Verification items for the finished model (mm, model axes). Face numbers are marked on the shaded views. A direction names the side the tool comes from. Round coordinates to 2 decimals unless told otherwise and drop trailing zeros. Write each loop counter-clockwise with the first axis right and the second up, starting at its lowest first coordinate (ties: lowest second). Pieces come first, ordered by that corner, then holes. Notation, with made-up numbers: (72.5, 87) -> (128.5, 87) arc R21 ccw to (128.5, 92) -> close; hole circle Ø2 at (9.5, 25). An arc over 180 degrees is marked (long way). Answer as a JSON object with one key per item and string values. Group by question number.
(1) Sectioned sample at A-A on x = 0. Record the cut outline in (y, z).
(2) Sectioned sample at B-B on z = 14.25. Record the cut outline in (x, y), and give its area (3 significant figures).
(3) Set-up check for the marked faces 1, 2, 3 and 4: record each of +Z, -Z, +X, -X, +Y, -Y from which the full face is reachable in a straight line by a thin tool's end or side.
(4) Gauge pin test, flat ends, axial feed: pin 1 Ø0.9 at (y, z) = (1, 23.5) entering from +X; pin 2 Ø2.5 at (x, y) = (0, 0) entering from +Z; pin 3 Ø1 at (x, z) = (-4, 18) entering from -Y. Record the tip position at first contact, or that the pin passes through.
(5) Sectioned sample at D-D on z = 5.25. Record the cut outline in (x, y), and give its area (3 significant figures).
(6) Scan lines: L1, parallel to X at y = 0, z = 16.75; L2, parallel to Z at x = -2.5, y = 6; L3, parallel to Y at x = -0.75, z = 12.75. Record each from-to range of solid material in increasing order. Write a range as from..to.
(7) Sectioned sample at C-C on y = 6.5. Record the cut outline in (x, z).
Solid Edge part; units mm, degrees
sketch "Sketch1" plane through (0, 0, 0) normal (0, 0, 1) x (1, 0, 0)
  circle A0 centre (0, 0) radius 15
extrude "Protrusion1" add sketch "Sketch1" along normal blind 10
sketch "Sketch2" plane through (0, 0, 10) normal (0, 0, 1) x (1, 0, 0)
  circle A0 centre (0, 0) radius 8
extrude "Extrusionsausprägung_2" add sketch "Sketch2" along normal blind 10
sketch "Sketch3" plane through (0, 0, 20) normal (0, 0, 1) x (1, 0, 0)
  circle A0 centre (0, 0) radius 6
extrude "Extrusionsausprägung_3" add sketch "Sketch3" along normal blind 2.5
sketch "Sketch4" plane through (0, 0, 22.5) normal (0, 0, 1) x (1, 0, 0)
  line L0 (-3.25, -3.25) -> (3.25, -3.25)
  line L1 (3.25, -3.25) -> (3.25, 3.25)
  line L2 (3.25, 3.25) -> (-3.25, 3.25)
  line L3 (-3.25, 3.25) -> (-3.25, -3.25)
extrude "Extrusionsausprägung_4" add sketch "Sketch4" along normal blind 3
sketch "Sketch5" plane through (0, 0, 10) normal (0, 0, 1) x (1, 0, 0)
  line L0 (-16.4348, 18.9803) -> (16.4348, 18.9803)
  line L1 (16.4348, 18.9803) -> (16.4348, -18.9803)
  line L2 (16.4348, -18.9803) -> (-16.4348, -18.9803)
  line L3 (-16.4348, -18.9803) -> (-16.4348, 18.9803)
  line L4 (-8, 16.4595) -> (8, 16.4595)
  line L5 (8, 16.4595) -> (8, -16.4595)
  line L6 (8, -16.4595) -> (-8, -16.4595)
  line L7 (-8, -16.4595) -> (-8, 16.4595)
  dimension "D1" = 8
extrude "Cutout1" cut sketch "Sketch5" against normal through all
hole "Bohrung_1" at (0, 0, 25.5) direction (0, 0, -1) diameter 3 depth 15
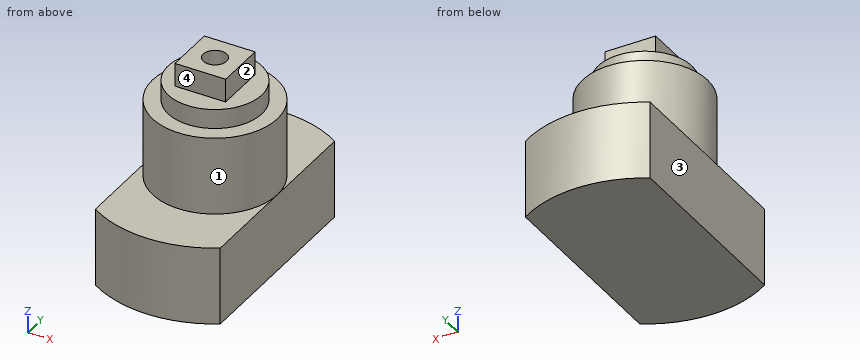
Computed values:
{
 "1": {"outline": "(-15, 0) -> (15, 0) -> (15, 10) -> (8, 10) -> (8, 20) -> (6, 20) -> (6, 22.5) -> (3.25, 22.5) -> (3.25, 25.5) -> (1.5, 25.5) -> (1.5, 10.5) -> (-1.5, 10.5) -> (-1.5, 25.5) -> (-3.25, 25.5) -> (-3.25, 22.5) -> (-6, 22.5) -> (-6, 20) -> (-8, 20) -> (-8, 10) -> (-15, 10) -> close"},
 "2": {"outline": "circle Ø16 at (0, 0); hole circle Ø3 at (0, 0)", "area": "194 mm2"},
 "3": {"face 1": "+Z", "face 2": "+Z, +X, +Y, -Y", "face 3": "+Z, -Z, -X, +Y, -Y", "face 4": "+Z, +X, -X, -Y"},
 "4": {"pin 1": "x = 3.25", "pin 2": "z = 10.5", "pin 3": "y = -7.19"},
 "5": {"outline": "(-8, -12.69) arc R15 ccw to (8, -12.69) -> (8, 12.69) arc R15 ccw to (-8, 12.69) -> close", "area": "456 mm2"},
 "6": {"L1": "-8..-1.5, 1.5..8", "L2": "0..20", "L3": "-7.96..-1.3, 1.3..7.96"},
 "7": {"outline": "(-8, 0) -> (8, 0) -> (8, 10) -> (4.66, 10) -> (4.66, 20) -> (-4.66, 20) -> (-4.66, 10) -> (-8, 10) -> close"}
}
